Design review of the part built by this model. Coordinates are the model's own, in mm. A direction names the side the tool comes from. Coordinates: 2 decimals unless noted, no trailing zeros. Write each loop counter-clockwise with the first axis right and the second up, starting at its lowest first coordinate (ties: lowest second). Pieces come first, ordered by that corner, then holes. Notation, with made-up numbers: (62.5, -27.5) - (89.5, -27.5) arc R29 ccw to (89.5, 6.5) - close; hole circle Ø3 at (70.25, 69.25). An arc over 180 degrees is marked (long way). Use a Markdown table: item, result.
from build123d import *

# Parameters (mm, degrees)
EXTRUDE_THIN1_DEPTH = 787.4
FILLET1_R           = 1.651


with BuildPart() as part:
    # Sketch1 → Extrude-Thin1 (new body)
    with BuildSketch(Plane.XY):
        with BuildLine():
            Line((0, 0), (-16.66875, 0))
            Line((-16.66875, 0), (-16.66875, 12.7))
            ThreePointArc((-16.66875, 12.7), (-29.102138, 17.386858), (-35.347799, 29.114922))
            ThreePointArc((-35.347799, 29.114922), (-46.618799, 50.279536), (-69.05625, 58.7375))
            Line((-69.05625, 58.7375), (-69.05625, 64.29375))
            Line((-69.05625, 64.29375), (-80.16875, 64.29375))
            Line((-80.16875, 64.29375), (-80.16875, 84.93125))
            Line((-80.16875, 84.93125), (-67.46875, 84.93125))
            Line((-67.46875, 84.93125), (-67.46875, 83.28025))
            Line((-67.46875, 83.28025), (-78.51775, 83.28025))
            Line((-78.51775, 83.28025), (-78.51775, 65.94475))
            Line((-78.51775, 65.94475), (-67.40525, 65.94475))
            Line((-67.40525, 65.94475), (-67.40525, 60.35024))
            ThreePointArc((-67.40525, 60.35024), (-44.915012, 50.967453), (-33.710486, 29.327071))
            ThreePointArc((-33.710486, 29.327071), (-27.378357, 18.096412), (-15.01775, 14.430495))
            Line((-15.01775, 14.430495), (-15.01775, 1.651))
            Line((-15.01775, 1.651), (0, 1.651))
            Line((0, 1.651), (0, 0))
        make_face()
    extrude(amount=-EXTRUDE_THIN1_DEPTH)

    # Fillet1
    fillet1_edges = [part.edges().sort_by_distance(p)[0] for p in [
        (-67.40525, 65.94475, -393.7),
        (-15.01775, 14.430495, -393.7),
        (-16.66875, 0, -393.7),
        (-69.05625, 58.7375, -393.7),
        (-80.16875, 64.29375, -393.7),
        (-80.16875, 84.93125, -393.7),
    ]]
    fillet(fillet1_edges, radius=FILLET1_R)


solid = part.part
(1) Take a section at A-A on z = -624.5. Write out the cut boundary in (x, y), and give its area (3 significant figures).
Determined:
| item | result |
|---|---|
| outline | (-80.17, 65.94) arc R1.65 ccw to (-78.52, 64.29) - (-69.06, 64.29) - (-69.06, 60.35) arc R1.65 ccw to (-67.48, 58.7) arc R33.99 cw to (-35.35, 29.11) arc R18.84 ccw to (-16.67, 12.7) - (-16.67, 1.65) arc R1.65 ccw to (-15.02, 0) - (0, 0) - (0, 1.65) - (-15.02, 1.65) - (-15.02, 12.7) arc R1.65 ccw to (-16.67, 14.35) arc R17.18 cw to (-33.71, 29.33) arc R35.64 ccw to (-67.41, 60.35) - (-67.41, 64.29) arc R1.65 ccw to (-69.06, 65.94) - (-78.52, 65.94) - (-78.52, 83.28) - (-67.47, 83.28) - (-67.47, 84.93) - (-78.52, 84.93) arc R1.65 ccw to (-80.17, 83.28) - close |
| area | 248 mm2 |
(2) For pin 1 (5.5 mm diameter, centred on x = -71, z = -398, fed in from -Y); pin 2 (4.5 mm diameter, centred on y = 63, z = -380.5, fed in from +X); pin 3 (10 mm diameter, centred on y = 54, z = -686, fed in from -X), all flat-tipped, find the tip position at first contact; note any pin that passes through.
Determined:
| item | result |
|---|---|
| pin 1 | y = 58.93 |
| pin 2 | x = -67.41 |
| pin 3 | x = -68.36 |
(3) Draft analysis for pull direction Y (two halves, no side actions). For faces 3 (the flat face through (-78.518, 75, -388)), 4 (the cylindrical face through (-29, 17.3, -388.2)), 5 (the cylindrical face through (-45.17, 51.2, -388.19)), 6 (the flat face through (-40, 43, 0)), state which applies: +Y half, -Y half, draft (parallel to the pull), parting line (faces both ways), or undercut.
Determined:
| item | result |
|---|---|
| face 3 | undercut |
| face 4 | -Y half |
| face 5 | +Y half |
| face 6 | draft |
(4) Take a section at B-B on y = 74. Write out the cut boundary in (x, z), and give its area (3 significant figures).
Determined:
| item | result |
|---|---|
| outline | (-80.17, -787.4) - (-78.52, -787.4) - (-78.52, 0) - (-80.17, 0) - close |
| area | 1,300 mm2 |
(5) For L1, parallel to X at y = 29, z = -302; L2, parallel to Y at x = -13, z = -519; L3, parallel to Y at x = -65.5, z = -201.5, list the stretches that pass through material, from the lowest coordinate up. Write a range as from..to.
Determined:
| item | result |
|---|---|
| L1 | -35.33..-33.66 |
| L2 | 0..1.65 |
| L3 | 58.55..60.21 |
(6) Take a section at C-C on x = -46.5. Write out the cut boundary in (y, z), and give its area (3 significant figures).
Determined:
| item | result |
|---|---|
| outline | (50.17, -787.4) - (52.34, -787.4) - (52.34, 0) - (50.17, 0) - close |
| area | 1,710 mm2 |
(7) Machinability: for faces 1 (the flat face through (-8, 1.651, -388)), 2 (the flat face through (-80.169, 74, -388)), which of the approach directions +Z, -Z, +X, -X, +Y, -Y give a long, thin tool a straight path to every point of the face, cutting with its end or side? Answer none if there is none.
Determined:
| item | result |
|---|---|
| face 1 | +Z, -Z, +X, +Y |
| face 2 | +Z, -Z, -X, +Y, -Y |
